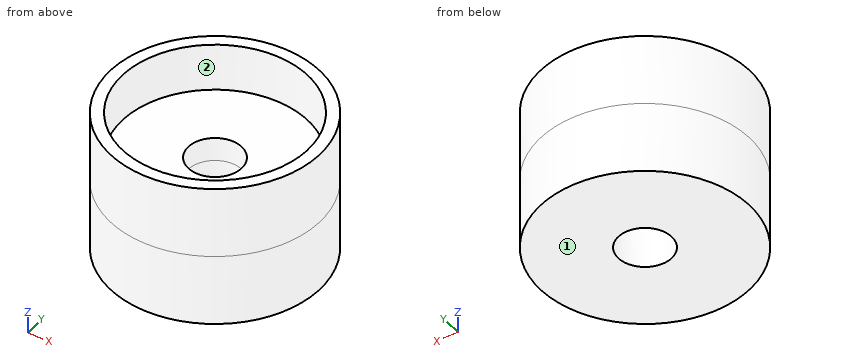
```python
from build123d import *

# Parameters (mm, degrees)
SKETCH1_R                = 4.40625
SKETCH1_R_2              = 3.90625
BOSS_EXTRUDE1_DEPTH      = 3
SKETCH1_3_R              = 4.40625
SKETCH1_3_R_2            = 3.90625
SKETCH1_3_R_3            = 1.125
BOSS_EXTRUDE2_DEPTH      = 1
BOSS_EXTRUDE2_DEPTH_BACK = 3


with BuildPart() as part:
    # Sketch1 → Boss-Extrude1 (new body)
    with BuildSketch(Plane.XY):
        Circle(SKETCH1_R)
        Circle(SKETCH1_R_2, mode=Mode.SUBTRACT)
    extrude(amount=BOSS_EXTRUDE1_DEPTH)

    # Sketch1_3 → Boss-Extrude2 (add, two sides)
    with BuildSketch(Plane.XY) as boss_extrude2_sk:
        Circle(SKETCH1_3_R)
        Circle(SKETCH1_3_R_2, mode=Mode.SUBTRACT)
        Circle(SKETCH1_3_R_2)
        Circle(SKETCH1_3_R_3, mode=Mode.SUBTRACT)
    extrude(amount=BOSS_EXTRUDE2_DEPTH)
    extrude(boss_extrude2_sk.sketch, amount=-BOSS_EXTRUDE2_DEPTH_BACK)


solid = part.part
```
Build history of the part. All positions in model axes, mm. Face numbers are marked on the shaded views. Coordinates: 2 decimals unless noted, no trailing zeros. Order: outer loops, then holes, each group sorted by start corner. A loop starts at its lowest first (then second) coordinate and runs counter-clockwise, first axis right, second up. Notation, with made-up numbers: (84.25, -6.75) -> (107.25, -6.75) arc R19 ccw to (107.25, 12.25) -> close; hole circle Ø3 at (89.25, 20.25). An arc over 180 degrees is marked (long way). Answer in a Markdown table with one row per item. Add a question column.
Q1. Drop flat-ended pins along their axis: pin 1 (1 mm diameter, centred on y = -3.5, z = 0, fed in from +X); pin 2 (1.5 mm diameter, centred on y = -1, z = 1.5, fed in from +X); pin 3 (4 mm diameter, centred on x = -1.5, y = 2.5, fed in from +Z); pin 4 (3 mm diameter, centred on x = -1.5, y = 0.5, fed in from +Z). Give the stop position or say it passes through.
Q2. Wall check: line 1 along Y through (x, z) = (0, -1) (3 decimals); line 2 along Z through (x, y) = (-1.5, -1.25); line 3 along Y through (x, z) = (0.5, -0.25). Give the ranges that are in metal, low to high. Write a range as [from, to].
Q3. Band-saw the part on A-A, the plane y = 0. List the corners of the cut face in (x, z) (3 decimals).
Q4. Mould opens along X. For the marked faces 1 and 2 say: +X half, -X half, draft (parallel to the pull), parting line (faces both ways), or undercut.
Q5. Band-saw the part on D-D, the plane x = 3. List the corners of the cut face in (y, z), then the cut area to 3 significant figures.
Answers follow:
| question | item | result |
|---|---|---|
| 1 | pin 1 | x = 3.23 |
| 1 | pin 2 | x = 4.4 |
| 1 | pin 3 | z = 3 |
| 1 | pin 4 | z = 1 |
| 2 | line 1 | [-4.406, -1.125], [1.125, 4.406] |
| 2 | line 2 | [-3, 1] |
| 2 | line 3 | [-4.38, -1.01], [1.01, 4.38] |
| 3 | outline | (-4.406, -3) -> (-1.125, -3) -> (-1.125, 1) -> (-3.906, 1) -> (-3.906, 3) -> (-4.406, 3) -> close; (1.125, -3) -> (4.406, -3) -> (4.406, 3) -> (3.906, 3) -> (3.906, 1) -> (1.125, 1) -> close |
| 4 | face 1 | draft |
| 4 | face 2 | undercut |
| 5 | outline | (-3.23, -3) -> (3.23, -3) -> (3.23, 3) -> (2.5, 3) -> (2.5, 1) -> (-2.5, 1) -> (-2.5, 3) -> (-3.23, 3) -> close |
| 5 | area | 28.7 mm^2 |
